Work out the finished part from the listing and answer in its coordinate system (mm). A direction names the side the tool comes from. Give positions to 0.01 mm unless a question says otherwise; leave off trailing zeros. Order: outer loops, then holes, each group sorted by start corner. A loop starts at its lowest first (then second) coordinate and runs counter-clockwise, first axis right, second up. Notation, with made-up numbers: (81.25, 3) - (135.25, 3) arc R35 ccw to (135.25, 42) - close; hole circle Ø4 at (31.5, 70). An arc over 180 degrees is marked (long way). Write each question's results on one line, items separated by ' | '.
Autodesk Fusion 360 part; units mm, degrees
sketch "Sketch1" plane through (0, 0, 0) normal (0, 0, 1) x (1, 0, 0)
  circle A0 centre (0, 0) radius 8
  circle A1 centre (0, 0) radius 4
  dimension "d1" = 16
  dimension "d2" = 8
extrude "Extrude1" add sketch "Sketch1" along normal blind 7.6
sketch "Sketch2" plane through (0, 0, 7.6) normal (0, 0, 1) x (-1, 0, 0)
  circle A0 centre (0, 0) radius 4
  circle A1 centre (0, 0) radius 8
  circle A2 centre (0, 0) radius 6
  dimension "d5" = 12
extrude "Extrude2" add sketch "Sketch2" along normal blind 11 contours A2
sketch "Sketch3" plane through (0, 0, 18.6) normal (0, 0, 1) x (-1, 0, 0)
  circle A0 centre (0, 0) radius 4
  circle A1 centre (0, 0) radius 6
  circle A2 centre (0, 0) radius 8
  dimension "d8" = 16
extrude "Extrude3" add sketch "Sketch3" along normal blind 1.2 contours A1 | A2
1. A cutting plane is placed at C-C, the plane z = 9.5. Write down the section's boundary in (x, y).
Answer list:
outline: circle Ø12 at (0, 0); hole circle Ø8 at (0, 0)
2. A tool of negligible diameter and unlimited length cuts with its end or side. For faces 1 (the face through (6, 0, 13)), 2 (the face through (-1.73, 7.81, 3.75)), from which of +Z, -Z, +X, -X, +Y, -Y can it reach the whole face along a straight path? Write none if from no direction.
Answer list:
face 1: none | face 2: +Z, -Z
3. Given P1, Ø5, axis at x = -1, y = 1, coming from the +Z side; P2, Ø4, axis at x = -4.5, z = 15.5, coming from the +Y side; P3, Ø1.5, axis at y = -0.5, z = 9.5, coming from the -X side; P4, Ø4, axis at x = 4, z = 14, coming from the -Y side, each flat-ended and moving along its own axis, determine where each tip first touches the part or whether it passes through.
Answer list:
P1: through | P2: y = 5.45 | P3: x = -6 | P4: y = -5.66
4. A cutting plane is placed at B-B, the plane y = 7.25. Write down the section's boundary in (x, z), then the cut area to 3 significant figures.
Answer list:
outline: (-3.38, 0) - (3.38, 0) - (3.38, 7.6) - (-3.38, 7.6) - close; (-3.38, 18.6) - (3.38, 18.6) - (3.38, 19.8) - (-3.38, 19.8) - close | area: 59.5 mm^2
5. A cutting plane is placed at A-A, the plane x = 6.25. Write down the section's boundary in (y, z).
Answer list:
outline: (-4.99, 0) - (4.99, 0) - (4.99, 7.6) - (-4.99, 7.6) - close; (-4.99, 18.6) - (4.99, 18.6) - (4.99, 19.8) - (-4.99, 19.8) - close
6. Straight lines are drawn through the part: line 1 (Z direction, x = -6.75, y = -2.25); line 2 (X direction, y = 0, z = 15). For each, find the intervals that lie inside material, in ascending order. Write a range as [from, to].
Answer list:
line 1: [0, 7.6], [18.6, 19.8] | line 2: [-6, -4], [4, 6]
7. Determine the mould class of faces 3 (the face through (2, -6, 18.6)), 4 (the face through (-4, -2, 0)), 5 (the face through (1.73, -7.81, 19.19)), 6 (the face through (-2, 6, 7.6)) for opening direction Z: +Z half, -Z half, draft (parallel to the pull), parting line (faces both ways), or undercut.
Answer list:
face 3: undercut | face 4: -Z half | face 5: draft | face 6: undercut
